Source: CAD feature listing. Evaluate the final solid. Frame: model axes, mm. Coordinates: 2 decimals unless noted, no trailing zeros. Order: outer loops, then holes, each group sorted by start corner. A loop starts at its lowest first (then second) coordinate and runs counter-clockwise, first axis right, second up.
```python
from build123d import *

# Parameters (mm, degrees)
BASE_EXTRUDE_DEPTH = 15.875
SKETCH2_R          = 6.746875
CUT_EXTRUDE1_DEPTH = 54.126241924
CHAMFER1_SIZE      = 0.381


with BuildPart() as part:
    # Sketch1 → Base-Extrude (new, symmetric)
    with BuildSketch(Plane(origin=(0, 0, 0), x_dir=(0, 0, -1), z_dir=(1, 0, 0))):
        with BuildLine():
            Line((16.618356424, 1.016), (43.688, 1.016))
            ThreePointArc((43.688, 1.016), (44.226815367, 1.239184633), (44.45, 1.778))
            Line((44.45, 1.778), (44.45, 22.225))
            ThreePointArc((44.45, 22.225), (43.52006403, 24.47006403), (41.275, 25.4))
            Line((41.275, 25.4), (-41.275, 25.4))
            ThreePointArc((-41.275, 25.4), (-43.52006403, 24.47006403), (-44.45, 22.225))
            Line((-44.45, 22.225), (-44.45, 1.778))
            ThreePointArc((-44.45, 1.778), (-44.226815367, 1.239184633), (-43.688, 1.016))
            Line((-43.688, 1.016), (-16.618356424, 1.016))
            ThreePointArc((-16.618356424, 1.016), (-16.109007152, 1.21124845), (-15.860680599, 1.69693617))
            ThreePointArc((-15.860680599, 1.69693617), (0, 15.9512), (15.860680599, 1.69693617))
            ThreePointArc((15.860680599, 1.69693617), (16.109007152, 1.21124845), (16.618356424, 1.016))
        make_face()
    extrude(amount=BASE_EXTRUDE_DEPTH, both=True)

    # Sketch2 → Cut-Extrude1 (cut, through all)
    with BuildSketch(Plane(origin=(0, 25.4, 0), x_dir=(-1, 0, 0), z_dir=(0, 1, 0))):
        with Locations(Location((0, 25.4, 0), (0, 0, 90))):
            Circle(SKETCH2_R)
        with Locations(Location((0, -25.4, 0), (0, 0, 90))):
            Circle(SKETCH2_R)
    extrude(amount=-CUT_EXTRUDE1_DEPTH, mode=Mode.SUBTRACT)

    # Chamfer1
    chamfer1_edges = [part.edges().sort_by_distance(p)[0] for p in [
        (0, 1.016, 18.653125),
        (0, 25.4, 18.653125),
        (0, 1.016, -32.146875),
        (0, 25.4, -32.146875),
    ]]
    chamfer(chamfer1_edges, length=CHAMFER1_SIZE)


solid = part.part
```
1. Pin query (flat end, axial travel): P1, Ø8, axis at x = 0, z = 25.4, coming from the -Y side. Return the tip coordinate at first contact, or that it passes through.
Findings:
P1: passes through
2. Section query D-D on y = 19.75. Return loops of the section in (x, z) (3 decimals).
Findings:
outline: (-15.875, -44.45) - (15.875, -44.45) - (15.875, 44.45) - (-15.875, 44.45) - close; hole circle Ø13.494 at (0, -25.4); hole circle Ø13.494 at (0, 25.4)
3. Section query C-C on x = 0. Return loops of the section in (y, z) (3 decimals).
Findings:
outline: (1.016, -43.688) arc R0.762 ccw to (1.778, -44.45) - (22.225, -44.45) arc R3.175 ccw to (25.4, -41.275) - (25.4, -32.528) - (25.019, -32.147) - (1.397, -32.147) - (1.016, -32.528) - close; (1.016, -18.272) - (1.397, -18.653) - (25.019, -18.653) - (25.4, -18.272) - (25.4, 18.272) - (25.019, 18.653) - (1.397, 18.653) - (1.016, 18.272) - (1.016, 16.618) arc R0.762 ccw to (1.697, 15.861) arc R15.951 cw to (1.697, -15.861) arc R0.762 ccw to (1.016, -16.618) - close; (1.016, 32.528) - (1.397, 32.147) - (25.019, 32.147) - (25.4, 32.528) - (25.4, 41.275) arc R3.175 ccw to (22.225, 44.45) - (1.778, 44.45) arc R0.762 ccw to (1.016, 43.688) - close
4. Draft query along Z for faces 1 (the face through (0, 12, -44.45)), 2 (the face through (-15.875, 16.1, 0.6)), 3 (the face through (-2.584, 13.373, 31.632)). Return one class per face: released by +Z, released by -Z, zero draft, split by the parting line, or undercut.
Findings:
face 1: released by -Z
face 2: zero draft
face 3: undercut
5. Section query B-B on y = 14. Return loops of the section in (x, z) (3 decimals), plus the area to 3 significant figures.
Findings:
outline: (-15.875, -44.45) - (15.875, -44.45) - (15.875, -7.645) - (-15.875, -7.645) - close; (-15.875, 7.645) - (15.875, 7.645) - (15.875, 44.45) - (-15.875, 44.45) - close; hole circle Ø13.494 at (0, -25.4); hole circle Ø13.494 at (0, 25.4)
area: 2,050 mm2
6. Section query A-A on z = 25.4. Return loops of the section in (x, y) (3 decimals).
Findings:
outline: (-15.875, 1.016) - (-7.128, 1.016) - (-6.747, 1.397) - (-6.747, 25.019) - (-7.128, 25.4) - (-15.875, 25.4) - close; (6.747, 1.397) - (7.128, 1.016) - (15.875, 1.016) - (15.875, 25.4) - (7.128, 25.4) - (6.747, 25.019) - close
7. Ray query, line 1 (X direction, y = 12, z = -25.5) (3 decimals); line 2 (Z direction, x = -4.5, y = 24.25); line 3 (Z direction, x = -3, y = 4). Return the intervals inside material, ascending.
Findings:
line 1: x = -15.875 to -6.746, 6.746 to 15.875
line 2: z = -43.72 to -30.43, -20.37 to 20.37, 30.43 to 43.72
line 3: z = -44.45 to -31.44, -19.36 to -15.44, 15.44 to 19.36, 31.44 to 44.45
